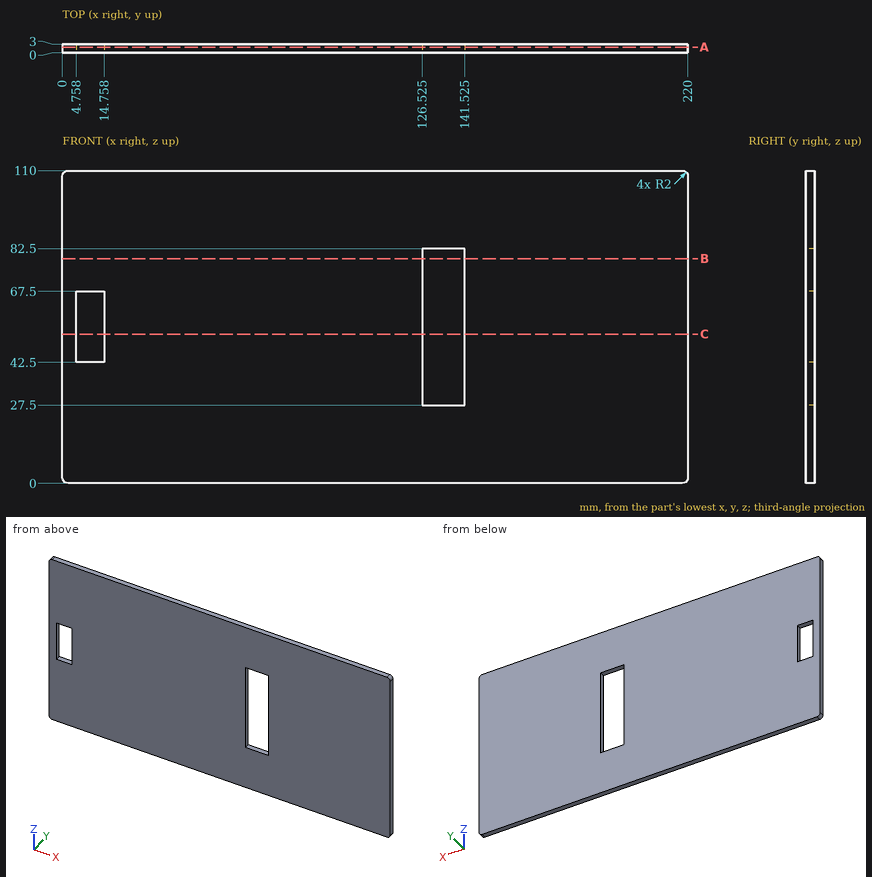
Print and shaded views of the part. All mm, measured from the part's lowest x, y and z. Coordinates: 2 decimals unless noted, no trailing zeros. Loops run counter-clockwise (first coordinate to the right, second up) from the corner with the lowest first, then second, coordinate; pieces in that order, holes last. Notation, with made-up numbers: (3.25, -0.75) - (12.25, -0.75) arc R9 ccw to (12.25, 16.25) - close; hole circle Ø6 at (-14.5, 59). An arc over 180 degrees is marked (long way). Use one line per item in the form item = value. Start each with the question number.
1) Drill centre lines: L1, parallel to X at y = 2.15, z = 32 (3 decimals); L2, parallel to X at y = 2.05, z = 54.5 (3 decimals); L3, parallel to Z at x = 137.5, y = 1.05. Where is each one in solid material? Low to high. Write a range as from..to.
2) Band-saw the part on A-A (y = 1.9). Give the cut face in (x, z) (3 decimals), and give its area (3 significant figures).
3) Band-saw the part on C-C (z = 52.5). Give the cut face in (x, y) (3 decimals), and give its area (3 significant figures).
4) Band-saw the part on B-B (z = 79). Give the cut face in (x, y) (3 decimals), and give its area (3 significant figures).
Check values:
q1.L1 = 0..126.525, 141.525..220
q1.L2 = 0..4.758, 14.758..126.525, 141.525..220
q1.L3 = 0..27.5, 82.5..110
q2.outline = (0, 2) arc R2 ccw to (2, 0) - (218, 0) arc R2 ccw to (220, 2) - (220, 108) arc R2 ccw to (218, 110) - (2, 110) arc R2 ccw to (0, 108) - close; hole (4.758, 42.5) - (14.758, 42.5) - (14.758, 67.5) - (4.758, 67.5) - close; hole (126.525, 27.5) - (141.525, 27.5) - (141.525, 82.5) - (126.525, 82.5) - close
q2.area = 23,100 mm2
q3.outline = (0, 0) - (4.758, 0) - (4.758, 3) - (0, 3) - close; (14.758, 0) - (126.525, 0) - (126.525, 3) - (14.758, 3) - close; (141.525, 0) - (220, 0) - (220, 3) - (141.525, 3) - close
q3.area = 585 mm2
q4.outline = (0, 0) - (126.525, 0) - (126.525, 3) - (0, 3) - close; (141.525, 0) - (220, 0) - (220, 3) - (141.525, 3) - close
q4.area = 615 mm2
